Autodesk Inventor part; units mm, degrees
ref_plane "YZ Plane" through (0, 0, 0) normal (1, 0, 0) x (0, 1, 0)
ref_plane "XZ Plane" through (0, 0, 0) normal (0, 1, 0) x (-1, 0, 0)
ref_plane "XY Plane" through (0, 0, 0) normal (0, 0, 1) x (1, 0, 0)
sketch "Sketch1" plane through (0, 0, 0) normal (0, 0, 1) x (1, 0, 0)
  line L0 (-10, -10) -> (10, -10)
  line L1 (10, -10) -> (10, 10)
  line L2 (10, 10) -> (-10, 10)
  line L3 (-10, 10) -> (-10, -10)
  line L4 (-10, -10) -> (10, 10) construction
  line L5 (10, -10) -> (-10, 10) construction
  circle A0 centre (0, 0) radius 2.4
  dimension "d0" = 20
  dimension "d1" = 20
  dimension "d2" = 4.8
extrude "Extrusion1" add sketch "Sketch1" along normal blind 2
chamfer "Chamfer1" distance 0.5 angle 45 4 edges at (10, 0, 0) (0, 10, 0) (-10, 0, 0) (0, -10, 0)
sketch "Sketch2" plane through (0, 0, 2) normal (0, 0, 1) x (1, 0, 0)
  line L0 (10, 10) -> (10, -10)
  line L1 (-10, -6) -> (10, -6)
  line L2 (10, -6) -> (10, 6)
  line L3 (10, 6) -> (-10, 6)
  line L4 (-10, 6) -> (-10, -6)
  line L5 (-10, -6) -> (10, 6) construction
  line L6 (10, -6) -> (-10, 6) construction
  point P0 (0, 0)
  point P1 (10, -6)
  dimension "d8" = 12
extrude "Extrusion2" add sketch "Sketch2" along normal blind 7
sketch "Sketch5" plane through (-10, -6, 2) normal (0, -1, 0) x (1, 0, 0)
  line L0 (20, 0) -> (0, 0)
  line L1 (4.5, 0) -> (15.5, 0)
  line L2 (15.5, 0) -> (15.5, 3)
  line L3 (15.5, 3) -> (4.5, 3)
  line L4 (4.5, 3) -> (4.5, 0)
  line L5 (0, 0) -> (0, 7)
  line L6 (20, 0) -> (20, 7)
  point P0 (10, -2)
  dimension "d18" = 3
  dimension "d19" = 4.5
  dimension "d20" = 4.5
extrude "Extrusion4" cut sketch "Sketch5" against normal through all
sketch "Sketch6" plane through (0, 0, 9) normal (0, 0, 1) x (1, 0, 0)
  circle A0 centre (0, 0) radius 2.4 construction
  circle A1 centre (0, 0) radius 4
  dimension "d23" = 8
extrude "Extrusion5" cut sketch "Sketch6" against normal up to surface (7 mm away)
chamfer "Chamfer4" distance 1.5 angle 45 2 edges at (-5.5, 0, 5) (5.5, 0, 5)
chamfer "Chamfer5" distance 1.5 angle 45 6 edges at (0, -6, 5) (0, 6, 5) (-4.75, -6, 4.25) (4.75, -6, 4.2501) (4.75, 6, 4.25) (-4.75, 6, 4.2501)
chamfer "Chamfer6" distance 1.5 angle 45 2 edges at (-10, 0, 9) (10, 0, 9)
chamfer "Chamfer7" distance 2 angle 45 8 edges at (10, 10, 1.25) (-10, 10, 1.25) (-10, -10, 1.25) (10, -10, 1.25) (7.75, -6, 2) (-7.75, -6, 2) (-7.75, 6, 2) (7.75, 6, 2)
equation "\"d20\" = d19"
properties part number "_3DPrint"
Input: part model. Units: mm. Frame: model coordinates. A direction names the side the tool comes from. Give positions to 0.01 mm unless a question says otherwise; leave off trailing zeros. Order: outer loops, then holes, each group sorted by start corner. A loop starts at its lowest first (then second) coordinate and runs counter-clockwise, first axis right, second up. Notation, with made-up numbers: M 38,81.5 L 88,81.5 A10 cw 88,91.5 Z; hole C -21,82.5 d5. An arc over 180 degrees is marked long. One line per question, with ' | ' between items. Start each with the question number.
1. Access query for faces 1 (the face through (5, 0, 4)), 2 (the face through (-4.851, 5.24, 5.195)), 3 (the face through (0, 6, 7)), 4 (the face through (-4.866, -5.261, 5.209)). Directions: +Z, -Z, +X, -X, +Y, -Y. A direction counts if a zero-diameter tool reaches every point of the face in a straight line with its end or side. Return the directions, or none.
2. Section query C-C (y = 4.25). Return the cut outline in (x, z).
3. First-contact query: pin 1 Ø6.5 at (x, y) = (0, 0) entering from +Z; pin 2 Ø3 at (y, z) = (7.5, 3.5) entering from -X; pin 3 Ø4.5 at (x, y) = (0, 0) entering from +Z; pin 4 Ø1.5 at (x, z) = (1.5, 6.5) entering from -Y. Flat tips, straight axial feed; report the tip coordinate or a pass-through.
4. Pull-direction query (Z, two-part tool) for faces 5 (the face through (3, 3, 5)), 6 (the face through (-0.867, -3.905, 7.028)), 7 (the face through (-2, 2, 0)), 8 (the face through (-9.3, 0.1, 8.2)); classes: released by +Z, released by -Z, zero draft, split by the parting line, or undercut.
5. Section query B-B (x = 0). Return the cut outline in (y, z).
6. Section query A-A (z = 3.25). Return the cut outline in (x, y).
7. Material intervals for probe 1 along X at (y, z) = (-4.75, 2.5); probe 2 along Z at (x, y) = (2, 4.25); probe 3 along Y at (x, z) = (0, 7.6), sorted ascending. Write a range as [from, to].
8. Section query D-D (z = 1.75). Return the cut outline in (x, y), and give its area (3 significant figures).
Here are the results:
1) face 1: +Y, -Y | face 2: +Y | face 3: +Z, +X, -X, +Y | face 4: -Y
2) outline: M -10,0.5 L -9.5,0 L 9.5,0 L 10,0.5 L 10,7.5 L 8.5,9 L -8.5,9 L -10,7.5 Z; hole M -5.5,2 L 5.5,2 L 5.5,3.5 L 4,5 L -4,5 L -5.5,3.5 Z
3) pin 1: z = 2 | pin 2: x = -10 | pin 3: through | pin 4: y = -6
4) face 5: undercut | face 6: zero draft | face 7: released by -Z | face 8: released by +Z
5) outline: M -10,0.5 L -9.5,0 L -2.4,0 L -2.4,2 L -10,2 Z; M -6,6.5 L -4.5,5 L -4,5 L -4,9 L -6,9 Z; M 2.4,0 L 9.5,0 L 10,0.5 L 10,2 L 2.4,2 Z; M 4,5 L 4.5,5 L 6,6.5 L 6,9 L 4,9 Z
6) outline: M -10,-6.75 L -5.5,-6.75 L -5.5,6.75 L -10,6.75 Z; M 5.5,-6.75 L 10,-6.75 L 10,6.75 L 5.5,6.75 Z
7) probe 1: [-10, -5.5], [5.5, 10] | probe 2: [0, 2], [5, 9] | probe 3: [-6, -4], [4, 6]
8) outline: M -10,-8 L -8,-10 L 8,-10 L 10,-8 L 10,8 L 8,10 L -8,10 L -10,8 Z; hole C 0,0 d4.8 | area: 374 mm²
